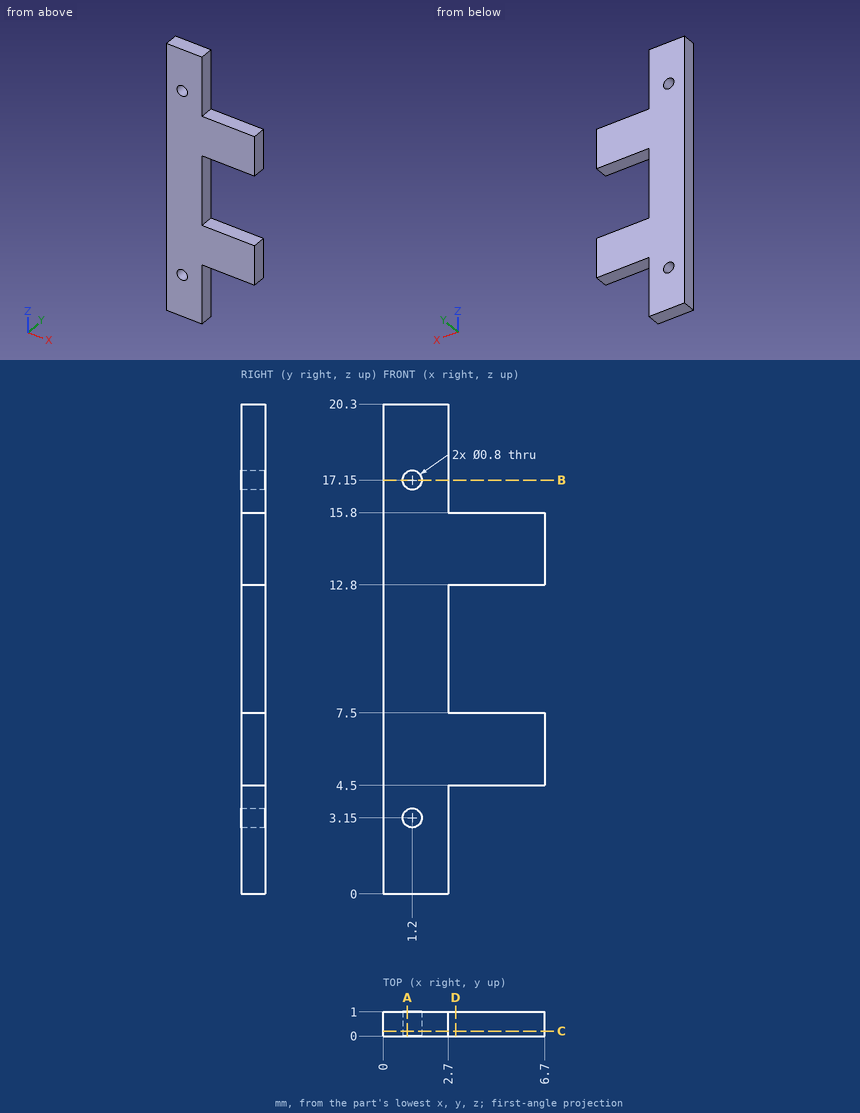
Here's the drawing with two shaded views (mm, measured from the low corner). I have some questions. Coordinates: 2 decimals unless noted, no trailing zeros. Loops run counter-clockwise (first coordinate to the right, second up) from the corner with the lowest first, then second, coordinate; pieces in that order, holes last.
Item 1: I'm going to push flat-ended pins straight in: pin 1 (0.5 mm diameter, centred on y = 0.5, z = 18, fed in from +X); pin 2 (1.5 mm diameter, centred on x = 4.5, z = 4, fed in from -Y). Where does each tip first touch, or does it pass through?
Answers below:
pin 1: stops at x = 2.7
pin 2: stops at y = 0
Item 2: Suppose I cut it at C-C (y = 0.2). Please give me the cut outline in (x, z), then the cut area to 3 significant figures.
Answers below:
outline: (0, 0) - (2.7, 0) - (2.7, 4.5) - (6.7, 4.5) - (6.7, 7.5) - (2.7, 7.5) - (2.7, 12.8) - (6.7, 12.8) - (6.7, 15.8) - (2.7, 15.8) - (2.7, 20.3) - (0, 20.3) - close; hole circle Ø0.8 at (1.2, 3.15); hole circle Ø0.8 at (1.2, 17.15)
area: 77.8 mm2
Item 3: Please list where these lines run through material, in increasing order: L1, parallel to Z at x = 1.25, y = 0.7; L2, parallel to X at y = 0.7, z = 17.15; L3, parallel to Z at x = 5, y = 0.15.
Answers below:
L1: z = 0 to 2.75, 3.55 to 16.75, 17.55 to 20.3
L2: x = 0 to 0.8, 1.6 to 2.7
L3: z = 4.5 to 7.5, 12.8 to 15.8
Item 4: Suppose I cut it at D-D (x = 3). Please give me the cut outline in (y, z).
Answers below:
outline: (0, 4.5) - (1, 4.5) - (1, 7.5) - (0, 7.5) - close; (0, 12.8) - (1, 12.8) - (1, 15.8) - (0, 15.8) - close
Item 5: Suppose I cut it at B-B (z = 17.15). Please give me the cut outline in (x, y), then the cut area to 3 significant figures.
Answers below:
outline: (0, 0) - (0.8, 0) - (0.8, 1) - (0, 1) - close; (1.6, 0) - (2.7, 0) - (2.7, 1) - (1.6, 1) - close
area: 1.90 mm2
Item 6: Suppose I cut it at A-A (x = 1). Please give me the cut outline in (y, z).
Answers below:
outline: (0, 0) - (1, 0) - (1, 2.8) - (0, 2.8) - close; (0, 3.5) - (1, 3.5) - (1, 16.8) - (0, 16.8) - close; (0, 17.5) - (1, 17.5) - (1, 20.3) - (0, 20.3) - close
